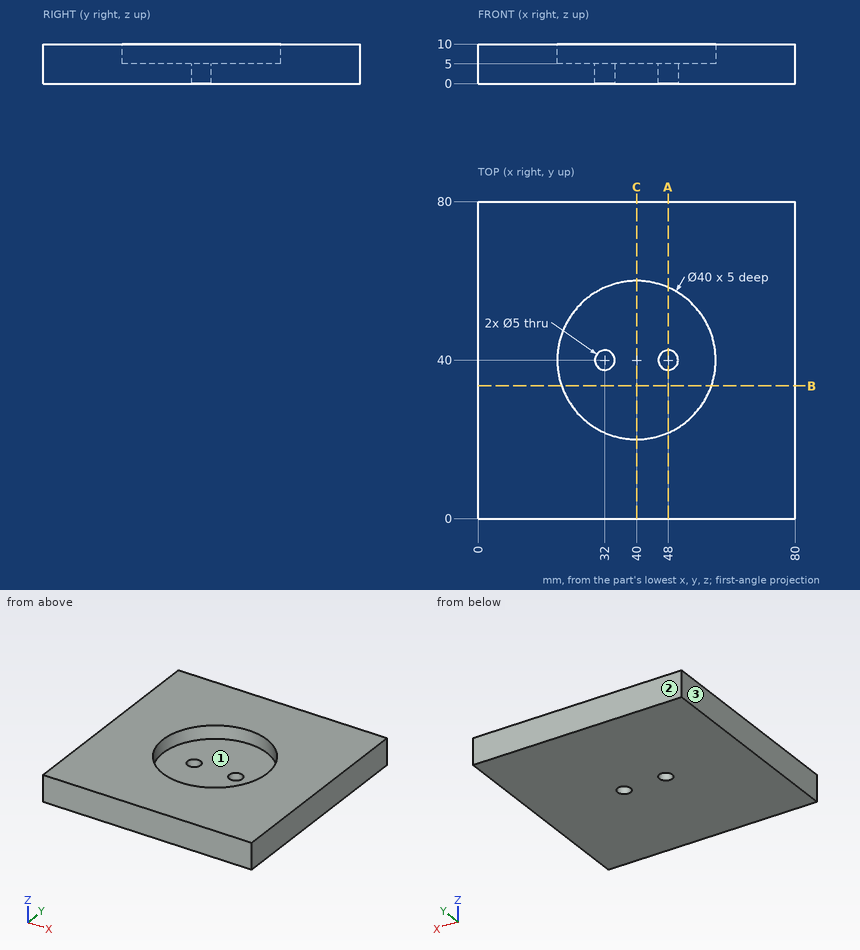
Job drawing, mm, ordinate dimensions from the low corner. One solid piece. Round coordinates to 2 decimals unless told otherwise and drop trailing zeros. Loops run counter-clockwise (first coordinate to the right, second up) from the corner with the lowest first, then second, coordinate; pieces in that order, holes last.
Item 1: Drop flat-ended pins along their axis: P1, Ø3, axis at x = 67, y = 56.5, coming from the -Z side; P2, Ø4.5, axis at x = 32, y = 40, coming from the -Z side; P3, Ø4, axis at x = 31.5, y = 27.5, coming from the +Z side. Give the stop position or say it passes through.
Item 2: Cut at B-B, the plane y = 33.5. Give the cut face in (x, z).
Item 3: Drill centre lines: line 1 (Y direction, x = 40, z = 7.3); line 2 (Y direction, x = 32, z = 3.6); line 3 (X direction, y = 38.5, z = 7.75). Where is each one in solid material? Low to high.
Item 4: Cut at C-C, the plane x = 40. Give the cut face in (y, z), then the cut area to 3 significant figures.
Item 5: Cut at A-A, the plane x = 48. Give the cut face in (y, z), then the cut area to 3 significant figures.
Item 6: Mould opens along X. For the marked faces 1, 2 and 3 say: +X half, -X half, draft (parallel to the pull), parting line (faces both ways), or undercut.
A:
1. P1: stops at z = 0
1. P2: passes through
1. P3: stops at z = 5
2. outline: (0, 0) - (80, 0) - (80, 10) - (58.91, 10) - (58.91, 5) - (21.09, 5) - (21.09, 10) - (0, 10) - close
3. line 1: y = 0 to 20, 60 to 80
3. line 2: y = 0 to 37.5, 42.5 to 80
3. line 3: x = 0 to 20.06, 59.94 to 80
4. outline: (0, 0) - (80, 0) - (80, 10) - (60, 10) - (60, 5) - (20, 5) - (20, 10) - (0, 10) - close
4. area: 600 mm2
5. outline: (0, 0) - (37.5, 0) - (37.5, 5) - (21.67, 5) - (21.67, 10) - (0, 10) - close; (42.5, 0) - (80, 0) - (80, 10) - (58.33, 10) - (58.33, 5) - (42.5, 5) - close
5. area: 592 mm2
6. face 1: undercut
6. face 2: draft
6. face 3: -X half
